```python
from build123d import *

# Parameters (mm, degrees)
CYLINDER009_R          = 36.5125
CYLINDER009_DEPTH      = 1066.8
CYLINDER009_ROLL_ANGLE = 90


with BuildPart() as part:
    # Cylinder009 → Cylinder009 (new body)
    with BuildSketch(Plane.XY):
        Circle(CYLINDER009_R)
    extrude(amount=CYLINDER009_DEPTH)


with BuildPart() as part_1:
    # Cylinder009 roll: moved
    add(part.part.rotate(Axis((0, 0, 0), (1, 0, 0)), CYLINDER009_ROLL_ANGLE))


with BuildPart() as part_2:
    # Cylinder009 placement: moved
    add(part_1.part.moved(Location((-766.4, 2199.64, -99.2001))))


solid = part_2.part
```
Input: part model. Units: mm. Frame: model coordinates. Give positions to 0.01 mm unless a question says otherwise; leave off trailing zeros. Write each loop counter-clockwise with the first axis right and the second up, starting at its lowest first coordinate (ties: lowest second). Pieces come first, ordered by that corner, then holes. Notation, with made-up numbers: (4.25, -31) - (8.25, -31) arc R29 cw to (8.25, -8) - close; hole circle Ø8 at (-26.5, 62.5). An arc over 180 degrees is marked (long way). Write item = value, one per line. Start each with the question number.
1. Section query B-B, the plane y = 1952. Output: boundary loops of the cut face in (x, z) (1 decimal).
2. Section query C-C, the plane x = -789. Output: boundary loops of the cut face in (y, z), then the cut area to 3 significant figures.
3. Ray query, L1, parallel to Z at x = -764, y = 1904; L2, parallel to Z at x = -763, y = 1736; L3, parallel to X at y = 1304.5, z = -99.5. Return the intervals inside material, ascending.
4. Section query A-A, the plane x = -739.5. Output: boundary loops of the cut face in (y, z), then the cut area to 3 significant figures.
5. First-contact query: pin 1 Ø10 at (x, y) = (-788.5, 1322.5) entering from -Z; pin 2 Ø10 at (y, z) = (1609, -122) entering from +X; pin 3 Ø3 at (y, z) = (1836.5, -81.5) entering from -X. Flat tips, straight axial feed; report the tip coordinate or a pass-through.
Check sheet entries:
q1.outline = circle Ø73 at (-766.4, -99.2)
q2.outline = (1132.84, -127.88) - (2199.64, -127.88) - (2199.64, -70.52) - (1132.84, -70.52) - close
q2.area = 61,200 mm2
q3.L1 = -135.63 to -62.77
q3.L2 = -135.55 to -62.85
q3.L3 = -802.91 to -729.89
q4.outline = (1132.84, -123.89) - (2199.64, -123.89) - (2199.64, -74.51) - (1132.84, -74.51) - close
q4.area = 52,700 mm2
q5.pin_1 = -131.46
q5.pin_2 = -734.52
q5.pin_3 = -799.12
